Source: CAD feature listing. Evaluate the final solid. Frame: model axes, mm. A direction names the side the tool comes from. Coordinates: 2 decimals unless noted, no trailing zeros. Loops run counter-clockwise (first coordinate to the right, second up) from the corner with the lowest first, then second, coordinate; pieces in that order, holes last. Notation, with made-up numbers: (8, 26.25) -> (64, 26.25) arc R14 ccw to (64, 42.25) -> close; hole circle Ø3 at (30.5, 51). An arc over 180 degrees is marked (long way). One line per question, with ' | ' between items. Start each with the question number.
```python
from build123d import *

# Parameters (mm, degrees)
SKETCH1_R           = 2.2098
BOSS_EXTRUDE1_DEPTH = 3.175
SKETCH2_R           = 3.1623
CUT_EXTRUDE3_DEPTH  = 1.27
SKETCH3_R           = 2.2098
BOSS_EXTRUDE2_DEPTH = 2.159
SKETCH4_W           = 1.524
SKETCH4_H           = 25.654
CUT_EXTRUDE4_DEPTH  = 1.397
SKETCH5_R           = 12.7
CUT_EXTRUDE5_DEPTH  = 2.54


with BuildPart() as part:
    # Sketch1 → Boss-Extrude1 (new body)
    with BuildSketch(Plane.XY):
        with BuildLine():
            Line((-50.8, -31.75), (50.8, -31.75))
            ThreePointArc((50.8, -31.75), (55.290128061, -29.890128061), (57.15, -25.4))
            Line((57.15, -25.4), (57.15, 25.4))
            ThreePointArc((57.15, 25.4), (55.290128061, 29.890128061), (50.8, 31.75))
            Line((50.8, 31.75), (-50.8, 31.75))
            ThreePointArc((-50.8, 31.75), (-55.290128061, 29.890128061), (-57.15, 25.4))
            Line((-57.15, 25.4), (-57.15, -25.4))
            ThreePointArc((-57.15, -25.4), (-55.290128061, -29.890128061), (-50.8, -31.75))
        make_face()
        with Locations((-50.8, -25.4)):
            Circle(SKETCH1_R, mode=Mode.SUBTRACT)
        with Locations((-38.1, -25.4)):
            Circle(SKETCH1_R, mode=Mode.SUBTRACT)
        with Locations(Location((-50.8, 25.4, 0), (0, 0, 180))):
            Circle(SKETCH1_R, mode=Mode.SUBTRACT)
        with Locations(Location((-38.1, 25.4, 0), (0, 0, 180))):
            Circle(SKETCH1_R, mode=Mode.SUBTRACT)
        with Locations((50.8, 25.4)):
            Circle(SKETCH1_R, mode=Mode.SUBTRACT)
        with Locations((38.1, 25.4)):
            Circle(SKETCH1_R, mode=Mode.SUBTRACT)
        with Locations(Location((50.8, -25.4, 0), (0, 0, 180))):
            Circle(SKETCH1_R, mode=Mode.SUBTRACT)
        with Locations(Location((38.1, -25.4, 0), (0, 0, 180))):
            Circle(SKETCH1_R, mode=Mode.SUBTRACT)
    extrude(amount=-BOSS_EXTRUDE1_DEPTH)

    # Sketch2 → Cut-Extrude3 (cut)
    with BuildSketch(Plane.XY):
        with BuildLine():
            Line((50.8, 30.7975), (-50.8, 30.7975))
            ThreePointArc((-50.8, 30.7975), (-54.616608851, 29.216608851), (-56.1975, 25.4))
            Line((-56.1975, 25.4), (-56.1975, -25.4))
            ThreePointArc((-56.1975, -25.4), (-54.616608851, -29.216608851), (-50.8, -30.7975))
            Line((-50.8, -30.7975), (50.8, -30.7975))
            ThreePointArc((50.8, -30.7975), (54.616608851, -29.216608851), (56.1975, -25.4))
            Line((56.1975, -25.4), (56.1975, 25.4))
            ThreePointArc((56.1975, 25.4), (54.616608851, 29.216608851), (50.8, 30.7975))
        make_face()
        with Locations((38.1, 25.4)):
            Circle(SKETCH2_R, mode=Mode.SUBTRACT)
        with Locations((50.8, 25.4)):
            Circle(SKETCH2_R, mode=Mode.SUBTRACT)
        with Locations((50.8, -25.4)):
            Circle(SKETCH2_R, mode=Mode.SUBTRACT)
        with Locations((38.1, -25.4)):
            Circle(SKETCH2_R, mode=Mode.SUBTRACT)
        with Locations((-38.1, -25.4)):
            Circle(SKETCH2_R, mode=Mode.SUBTRACT)
        with Locations((-50.8, -25.4)):
            Circle(SKETCH2_R, mode=Mode.SUBTRACT)
        with Locations((-38.1, 25.4)):
            Circle(SKETCH2_R, mode=Mode.SUBTRACT)
        with Locations((-50.8, 25.4)):
            Circle(SKETCH2_R, mode=Mode.SUBTRACT)
    extrude(amount=-CUT_EXTRUDE3_DEPTH, mode=Mode.SUBTRACT)

    # Sketch3 → Boss-Extrude2 (add)
    with BuildSketch(Plane(origin=(0, 0, -3.175), x_dir=(-1, 0, 0), z_dir=(0, 0, -1))):
        with BuildLine():
            Line((-57.15, 25.4), (-57.15, -25.4))
            ThreePointArc((-57.15, -25.4), (-55.290128061, -29.890128061), (-50.8, -31.75))
            Line((-50.8, -31.75), (50.8, -31.75))
            ThreePointArc((50.8, -31.75), (55.290128061, -29.890128061), (57.15, -25.4))
            Line((57.15, -25.4), (57.15, 25.4))
            ThreePointArc((57.15, 25.4), (55.290128061, 29.890128061), (50.8, 31.75))
            Line((50.8, 31.75), (-50.8, 31.75))
            ThreePointArc((-50.8, 31.75), (-55.290128061, 29.890128061), (-57.15, 25.4))
        make_face()
        with Locations((-50.8, -25.4)):
            Circle(SKETCH3_R, mode=Mode.SUBTRACT)
        with Locations((-38.1, -25.4)):
            Circle(SKETCH3_R, mode=Mode.SUBTRACT)
        with Locations(Location((38.1, -25.4, 0), (0, 0, 180))):
            Circle(SKETCH3_R, mode=Mode.SUBTRACT)
        with Locations(Location((50.8, -25.4, 0), (0, 0, 180))):
            Circle(SKETCH3_R, mode=Mode.SUBTRACT)
        with Locations((50.8, 25.4)):
            Circle(SKETCH3_R, mode=Mode.SUBTRACT)
        with Locations((38.1, 25.4)):
            Circle(SKETCH3_R, mode=Mode.SUBTRACT)
        with Locations(Location((-38.1, 25.4, 0), (0, 0, 180))):
            Circle(SKETCH3_R, mode=Mode.SUBTRACT)
        with Locations(Location((-50.8, 25.4, 0), (0, 0, 180))):
            Circle(SKETCH3_R, mode=Mode.SUBTRACT)
    extrude(amount=BOSS_EXTRUDE2_DEPTH)

    # Sketch4 → Cut-Extrude4 (cut)
    with BuildSketch(Plane(origin=(57.15, 0, 0), x_dir=(0, 0, -1), z_dir=(1, 0, 0))):
        with Locations((2.667, 0)):
            Rectangle(SKETCH4_W, SKETCH4_H)
    cut_extrude4 = extrude(amount=-CUT_EXTRUDE4_DEPTH, mode=Mode.SUBTRACT)

    # Mirror1: Cut-Extrude4 across plane
    add(cut_extrude4.mirror(Plane(origin=(0, 0, 0), x_dir=(0, 0, 1), z_dir=(1, 0, 0))), mode=Mode.SUBTRACT)

    # Sketch5 → Cut-Extrude5 (cut)
    with BuildSketch(Plane(origin=(0, 0, -5.334), x_dir=(-1, 0, 0), z_dir=(0, 0, -1))):
        Circle(SKETCH5_R)
    extrude(amount=-CUT_EXTRUDE5_DEPTH, mode=Mode.SUBTRACT)


solid = part.part
```
(1) Cut plane C-C, the plane x = 0. Return the cut outline in (y, z), and give its area (3 significant figures).
(2) Contact query for flat-ended pins moving along their axis: pin 1 Ø0.5 at (y, z) = (6, -2.5) entering from +X; pin 2 Ø2.5 at (x, y) = (50.8, -25.4) entering from +Z; pin 3 Ø5 at (x, y) = (31, -21) entering from +Z; pin 4 Ø1.5 at (x, z) = (-56.5, -3) entering from +Y. Output: stop coordinate, or through.
(3) Access query for faces 4 (the cylindrical face through (48.291, 23.476, -0.626)), 5 (the flat face through (1, -31.75, -3)), 6 (the cylindrical face through (2.75, -12.4, -4.08)). Directions: +Z, -Z, +X, -X, +Y, -Y. A direction counts if a zero-diameter tool reaches every point of the face in a straight line with its end or side. Return the directions, or none.
(4) Ray query, L1, parallel to X at y = 25.4, z = -4.3; L2, parallel to Y at x = -50.8, z = -1.8. Return the intervals inside material, ascending.
(5) Draft query along X for faces 1 (the cylindrical face through (-55.24, -29.94, -2.63)), 2 (the cylindrical face through (-53.309, 23.476, -0.626)), 3 (the flat face through (-50, -23, 0)). Return one class per face: pulls with the +X half, pulls with the -X half, needs draft (parallel to the pull), parting line crosses it, or undercut.
(6) Cut plane A-A, the plane x = 38.1. Return the cut outline in (y, z), and give its area (3 significant figures).
Here are the results:
1) outline: (-31.75, -5.33) -> (-12.7, -5.33) -> (-12.7, -2.79) -> (12.7, -2.79) -> (12.7, -5.33) -> (31.75, -5.33) -> (31.75, 0) -> (30.8, 0) -> (30.8, -1.27) -> (-30.8, -1.27) -> (-30.8, 0) -> (-31.75, 0) -> close | area: 196 mm2
2) pin 1: stops at x = 55.75 | pin 2: passes through | pin 3: stops at z = -1.27 | pin 4: stops at y = 29.38
3) face 4: +Z | face 5: +Z, -Z, +X, -X, -Y | face 6: -Z
4) L1: x = -57.15 to -53.01, -48.59 to -40.31, -35.89 to 35.89, 40.31 to 48.59, 53.01 to 57.15 | L2: y = -31.75 to -27.61, -23.19 to 23.19, 27.61 to 31.75
5) face 1: pulls with the -X half | face 2: undercut | face 3: needs draft
6) outline: (-31.75, -5.33) -> (-27.61, -5.33) -> (-27.61, 0) -> (-28.56, 0) -> (-28.56, -1.27) -> (-30.8, -1.27) -> (-30.8, 0) -> (-31.75, 0) -> close; (-23.19, -5.33) -> (23.19, -5.33) -> (23.19, 0) -> (22.24, 0) -> (22.24, -1.27) -> (-22.24, -1.27) -> (-22.24, 0) -> (-23.19, 0) -> close; (27.61, -5.33) -> (31.75, -5.33) -> (31.75, 0) -> (30.8, 0) -> (30.8, -1.27) -> (28.56, -1.27) -> (28.56, 0) -> (27.61, 0) -> close | area: 229 mm2
